```python
from build123d import *

# Parameters (mm, degrees)
CROQUIS1_W              = 100
CROQUIS1_H              = 100
SALIENTE_EXTRUIR1_DEPTH = 12.5
CROQUIS2_R              = 35.5
CORTAR_EXTRUIR1_DEPTH   = 10
CROQUIS3_R              = 25.5
CORTAR_EXTRUIR2_DEPTH   = 72.414284285
CORTAR_EXTRUIR3_DEPTH   = 72.807033082
MATRIZC1_COUNT          = 4


with BuildPart() as part:
    # Croquis1 → Saliente-Extruir1 (new body)
    with BuildSketch(Plane(origin=(0, 0, 0), x_dir=(1, 0, 0), z_dir=(0, 1, 0))):
        Rectangle(CROQUIS1_W, CROQUIS1_H)
    extrude(amount=SALIENTE_EXTRUIR1_DEPTH)

    # Croquis2 → Cortar-Extruir1 (cut)
    with BuildSketch(Plane(origin=(0, 12.5, 0), x_dir=(1, 0, 0), z_dir=(0, 1, 0))):
        with Locations(Location((0, 0, 0), (0, 0, 270))):
            Circle(CROQUIS2_R)
    extrude(amount=-CORTAR_EXTRUIR1_DEPTH, mode=Mode.SUBTRACT)

    # Croquis3 → Cortar-Extruir2 (cut, through all)
    with BuildSketch(Plane(origin=(0, 2.5, 0), x_dir=(1, 0, 0), z_dir=(0, 1, 0))):
        with Locations(Location((0, 0, 0), (0, 0, 270))):
            Circle(CROQUIS3_R)
    extrude(amount=-CORTAR_EXTRUIR2_DEPTH, mode=Mode.SUBTRACT)

    # Croquis4 → Cortar-Extruir3 (cut, through all)
    with BuildSketch(Plane(origin=(0, 12.5, 0), x_dir=(1, 0, 0), z_dir=(0, 1, 0))):
        with BuildLine():
            ThreePointArc((36.75, 40), (37.701902961, 37.701902961), (40, 36.75))
            Line((40, 36.75), (40, 40))
            Line((40, 40), (36.75, 40))
        make_face()
        with BuildLine():
            Line((40, 40), (40, 36.75))
            ThreePointArc((40, 36.75), (42.298097039, 37.701902961), (43.25, 40))
            ThreePointArc((43.25, 40), (40, 43.25), (36.75, 40))
            Line((36.75, 40), (40, 40))
        make_face()
    cortar_extruir3 = extrude(amount=-CORTAR_EXTRUIR3_DEPTH, mode=Mode.SUBTRACT)

    # MatrizC1: Cortar-Extruir3 ×4 about axis
    matrizc1_axis = Axis((0, 0, 0), (0, 1, 0))
    for i in range(1, MATRIZC1_COUNT):
        add(cortar_extruir3.rotate(matrizc1_axis, i * 360 / MATRIZC1_COUNT), mode=Mode.SUBTRACT)


solid = part.part
```
Part model, mm, in its own coordinate system. Round coordinates to 2 decimals unless told otherwise and drop trailing zeros. Write each loop counter-clockwise with the first axis right and the second up, starting at its lowest first coordinate (ties: lowest second). Pieces come first, ordered by that corner, then holes. Notation, with made-up numbers: M 62.5,76 L 93.5,76 A10 cw 93.5,95 Z; hole C -6,-27.5 d3. An arc over 180 degrees is marked long. Answer as CSV lines item,"result". Start each with the question number.
1) Band-saw the part on D-D (z = 38). List the corners of the cut face in (x, y), then the cut area to 3 significant figures.
2) Band-saw the part on C-C (z = -13). List the corners of the cut face in (x, y), then the cut area to 3 significant figures.
3) Band-saw the part on B-B (y = 5.5). List the corners of the cut face in (x, z), then the cut area to 3 significant figures.
4) Band-saw the part on A-A (x = 0). List the corners of the cut face in (y, z).
5) Mould opens along Z. For faces 1 (the face through (-31.495, 7.57, 16.381)), 2 (the face through (-12, 0, -23)), 3 (the face through (-23, 2.5, 15)), 4 (the face through (-1, 6, -50)) say: +Z half, -Z half, draft (parallel to the pull), parting line (faces both ways), or undercut.
6) Drill centre lines: L1, parallel to X at y = 6.5, z = 0; L2, parallel to Z at x = 40.5, y = 0.75; L3, parallel to X at y = 0.6, z = 0. Where is each one in solid material? Low to high.
Worked out:
1,outline,"M -50,0 L -42.56,0 L -42.56,12.5 L -50,12.5 Z; M -37.44,0 L 37.44,0 L 37.44,12.5 L -37.44,12.5 Z; M 42.56,0 L 50,0 L 50,12.5 L 42.56,12.5 Z"
1,area,"1,120 mm²"
2,outline,"M -50,0 L -21.94,0 L -21.94,2.5 L -33.03,2.5 L -33.03,12.5 L -50,12.5 Z; M 21.94,0 L 50,0 L 50,12.5 L 33.03,12.5 L 33.03,2.5 L 21.94,2.5 Z"
2,area,"480 mm²"
3,outline,"M -50,-50 L 50,-50 L 50,50 L -50,50 Z; hole C -40,-40 d6.5; hole C -40,40 d6.5; hole C 0,0 d71; hole C 40,-40 d6.5; hole C 40,40 d6.5"
3,area,"5,910 mm²"
4,outline,"M 0,-50 L 12.5,-50 L 12.5,-35.5 L 2.5,-35.5 L 2.5,-25.5 L 0,-25.5 Z; M 0,25.5 L 2.5,25.5 L 2.5,35.5 L 12.5,35.5 L 12.5,50 L 0,50 Z"
5,face 1,"undercut"
5,face 2,"draft"
5,face 3,"undercut"
5,face 4,"-Z half"
6,L1,"-50 to -35.5, 35.5 to 50"
6,L2,"-50 to -43.21, -36.79 to 36.79, 43.21 to 50"
6,L3,"-50 to -25.5, 25.5 to 50"
